Geometry check sheet. Reference: the model listing, model coordinates, mm. Face numbers are marked on the shaded views. Coordinates: 2 decimals unless noted, no trailing zeros. Write each loop counter-clockwise with the first axis right and the second up, starting at its lowest first coordinate (ties: lowest second). Pieces come first, ordered by that corner, then holes. Notation, with made-up numbers: (27, 48.25) -> (62, 48.25) arc R18 cw to (62, 57.25) -> close; hole circle Ø11 at (-33, 32). An arc over 180 degrees is marked (long way). Answer in a Markdown table with one row per item. Add a question column.
Q1. Thickness scan on line 1 (Y direction, x = 0, z = 12.6); line 2 (Y direction, x = 19, z = 12.5); line 3 (X direction, y = 10, z = 10). Record the ranges inside material, lowest first.
Q2. Gauge pin test, flat ends, axial feed: P1, Ø3, axis at x = -32, y = 15, coming from the -Z side; P2, Ø3, axis at x = -32, y = 27, coming from the +Z side; P3, Ø2, axis at y = -18.5, z = 5, coming from the -X side. Record the tip position at first contact, or that the pin passes through.
Q3. Release check for a two-part mould opening along X. For the marked faces 1 and 2 record: pulls with the +X half, pulls with the -X half, needs draft (parallel to the pull), parting line crosses it, or undercut.
Q4. Section check C-C, the plane z = 5.5. Record the boundary of the cut face in (x, y).
Q5. Section check A-A, the plane y = 0. Record the boundary of the cut face in (x, z).
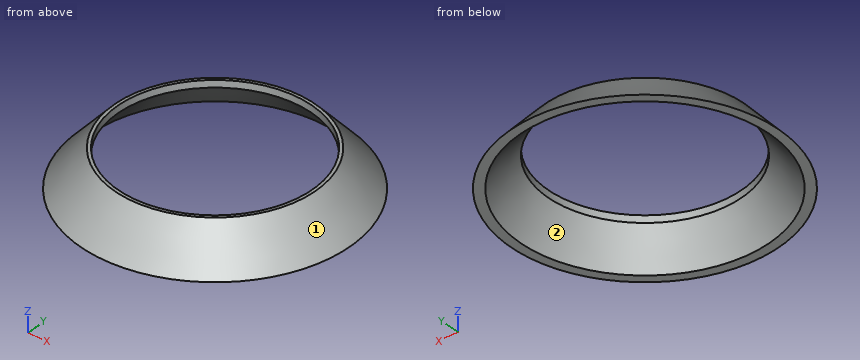
```python
from build123d import *

# Parameters (mm, degrees)
F2_T     = -2.5
F3_DEPTH = 25
F4_DEPTH = 25
F5_DEPTH = 27.501


with BuildPart() as f1:
    # F0 (on Front) → F1 (revolve)
    with BuildSketch(Plane.XZ):
        Polygon((0, 0), (0, 13.29), (-35, 13.29), (-46.9663697487, 0), align=None)
    revolve(axis=Axis((0, 0, 32.7267305849), (0, 0, 1)))

    # F2
    f2_openings = [f1.faces().sort_by_distance(p)[0] for p in [
        (0, 0, 0),
    ]]
    offset(amount=F2_T, openings=f2_openings)

    # F3 (add): a face of the model
    f3_faces = [f1.faces().sort_by_distance(p)[0] for p in [
        (0, 0, 10.79),
    ]]
    extrude(f3_faces, amount=F3_DEPTH)

    # F4 (add): a face of the model
    f4_faces = [f1.faces().sort_by_distance(p)[0] for p in [
        (0, 0, -14.21),
    ]]
    extrude(f4_faces, amount=-F4_DEPTH)

    # F5 (cut, through all): a face of the model
    f5_faces = [f1.faces().sort_by_distance(p)[0] for p in [
        (0, 0, -14.21),
    ]]
    extrude(f5_faces, amount=-F5_DEPTH, mode=Mode.SUBTRACT)


solid = f1.part
```
Calculated:
| question | item | result |
|---|---|---|
| 1 | line 1 | y = -35.62 to -33.89, 33.89 to 35.62 |
| 1 | line 2 | y = -30.24 to -28.06, 28.06 to 30.24 |
| 1 | line 3 | x = -36.62 to -33.12, 33.12 to 36.62 |
| 2 | P1 | stops at z = 7.51 |
| 2 | P2 | stops at z = 7.33 |
| 2 | P3 | stops at x = -39.32 |
| 3 | face 1 | parting line crosses it |
| 3 | face 2 | undercut |
| 4 | outline | circle Ø84.03 at (0, 0); hole circle Ø77.3 at (0, 0) |
| 5 | outline | (-46.97, 0) -> (-43.6, 0) -> (-33.89, 10.79) -> (-33.89, 13.29) -> (-35, 13.29) -> close; (33.89, 10.79) -> (43.6, 0) -> (46.97, 0) -> (35, 13.29) -> (33.89, 13.29) -> close |
